Autodesk Inventor part; units mm, degrees
ref_plane "YZ Plane" through (0, 0, 0) normal (1, 0, 0) x (0, 1, 0)
ref_plane "XZ Plane" through (0, 0, 0) normal (0, 1, 0) x (-1, 0, 0)
ref_plane "XY Plane" through (0, 0, 0) normal (0, 0, 1) x (1, 0, 0)
sketch "Sketch1" plane through (0, 0, 0) normal (1, 0, 0) x (0, 1, 0)
  line L0 (0, 0) -> (120, 0)
  line L1 (100, -61.25) -> (95, -61.25)
  line L2 (95, -61.25) -> (95, -110)
  line L3 (95, -110) -> (0, -110)
  line L4 (0, -110) -> (0, -135)
  line L5 (0, -135) -> (10, -135)
  line L6 (10, -135) -> (10, -115)
  line L7 (10, -115) -> (100, -115)
  line L8 (100, -115) -> (100, -61.25)
  line L9 (0, -114) -> (2, -114)
  line L10 (2, -114) -> (2, -117)
  line L11 (2, -117) -> (0, -117)
  line L12 (0, -117) -> (0, -114)
  dimension "d1" = 270
  dimension "d2" = 220
  dimension "d3" = 230
  dimension "d4" = 122.5
  dimension "d5" = 10
  dimension "d6" = 5
  dimension "d7" = 100
  dimension "d21" = 228
  dimension "d22" = 3
  dimension "d24" = 2
revolve "Revolution1" add sketch "Sketch1" angle 360 about axis through (0, 0, 0) along (0, 1, 0) contours L8 L7 L6 L5 L4 L11 L10 L9 L3 L2 L1
sketch "Sketch2" plane through (0, 10, 0) normal (0, 1, 0) x (1, 0, 0)
  point P0 (0, 0)
  point P1 (0, 125)
  point P2 (-73.4732, 101.1271)
  point P3 (-118.8821, 38.6271)
  point P4 (-118.8821, -38.6271)
  point P5 (-73.4732, -101.1271)
  point P6 (0, -125)
  point P7 (73.4732, -101.1271)
  point P8 (118.8821, -38.6271)
  point P9 (118.8821, 38.6271)
  point P10 (73.4732, 101.1271)
  dimension "d9" = 125
  dimension "d12" = 360
hole "Hole1" at (0, 10, -125) at (-73.4732, 10, -101.1271) at (-118.8821, 10, -38.6271) at (-118.8821, 10, 38.6271) at (-73.4732, 10, 101.1271) at (0, 10, 125) at (73.4732, 10, 101.1271) at (118.8821, 10, 38.6271) at (118.8821, 10, -38.6271) at (73.4732, 10, -101.1271) direction (0, -1, 0) diameter 5.9 end through all counterbore diameter 10.2 counterbore depth 1.2
properties part number "Vibrometer Housing"
Read the model definition and answer for the solid it produces. Units are mm, in the model's axes. A direction names the side the tool comes from. Coordinates: 2 decimals unless noted, no trailing zeros. Write each loop counter-clockwise with the first axis right and the second up, starting at its lowest first coordinate (ties: lowest second). Pieces come first, ordered by that corner, then holes. Notation, with made-up numbers: (-21.5, -27.75) -> (-13.5, -27.75) arc R29 ccw to (-13.5, -6.75) -> close; hole circle Ø5 at (45.25, 17). An arc over 180 degrees is marked (long way). Return JSON: item names as keys, results as strings.
(1) Which of the six approach directions +Z, -Z, +X, -X, +Y, -Y give full straight-line access (tool end or side, diameter ignored) to faces 3 (the cylindrical face through (-59.793, 97.465, 13.278)), 4 (the flat face through (-71, 8.8, -99)), 5 (the cylindrical face through (43.66, 1.01, -105.31))?
Answers below:
{"face 3": "+Y, -Y", "face 4": "+Y", "face 5": "-Y"}
(2) The part is cut by section B-B on y = 42. Give the vertices of the cut face in (x, z).
Answers below:
{"outline": "circle Ø230 at (0, 0); hole circle Ø220 at (0, 0)"}
(3) The part is cut by section C-C on x = -55.5. Give the vertices of the cut face in (y, z).
Answers below:
{"outline": "(0, -123.06) -> (10, -123.06) -> (10, -100.72) -> (100, -100.72) -> (100, -25.91) -> (95, -25.91) -> (95, -94.97) -> (0, -94.97) -> (0, -99.58) -> (2, -99.58) -> (2, -103) -> (0, -103) -> close; (0, 94.97) -> (95, 94.97) -> (95, 25.91) -> (100, 25.91) -> (100, 100.72) -> (10, 100.72) -> (10, 123.06) -> (0, 123.06) -> (0, 103) -> (2, 103) -> (2, 99.58) -> (0, 99.58) -> close"}
(4) Consider line 1 along Z through (x, y) = (3, 46); line 2 along Z through (x, y) = (0, 98.9); line 3 along Y through (x, z) = (40.5, -117). Determine where each line is inside the solid, lowest interval first. Write a range as from..to.
Answers below:
{"line 1": "-114.96..-109.96, 109.96..114.96", "line 2": "-115..-61.25, 61.25..115", "line 3": "0..10"}
(5) Each of these flat-tipped pins is pushed along its axis until it touches: P1, Ø4, axis at y = 55.5, z = 31.5, coming from the +X side; P2, Ø13.5, axis at x = -73.47, z = 101.13, coming from the +Y side; P3, Ø4, axis at y = 31, z = -10.5, coming from the -X side. Where does it stop, or does it pass through?
Answers below:
{"P1": "x = 111.15", "P2": "y = 10", "P3": "x = -114.69"}
(6) For a pull along X with two mould halves and no side action, classify faces 1 (the flat face through (109, 10, -39)), 2 (the cylindrical face through (77.998, 9.392, -98.774)) as pulls with the +X half, pulls with the -X half, needs draft (parallel to the pull), parting line crosses it, or undercut.
Answers below:
{"face 1": "needs draft", "face 2": "undercut"}
(7) The part is cut by section A-A on z = 0. Give the vertices of the cut face in (x, y).
Answers below:
{"outline": "(-135, 0) -> (-117, 0) -> (-117, 2) -> (-114, 2) -> (-114, 0) -> (-110, 0) -> (-110, 95) -> (-61.25, 95) -> (-61.25, 100) -> (-115, 100) -> (-115, 10) -> (-135, 10) -> close; (61.25, 95) -> (110, 95) -> (110, 0) -> (114, 0) -> (114, 2) -> (117, 2) -> (117, 0) -> (135, 0) -> (135, 10) -> (115, 10) -> (115, 100) -> (61.25, 100) -> close"}
(8) The part is cut by section D-D on z = -77.5. Give the vertices of the cut face in (x, y), then the cut area to 3 significant figures.
Answers below:
{"outline": "(-110.54, 0) -> (-87.65, 0) -> (-87.65, 2) -> (-83.6, 2) -> (-83.6, 0) -> (-78.06, 0) -> (-78.06, 95) -> (78.06, 95) -> (78.06, 0) -> (83.6, 0) -> (83.6, 2) -> (87.65, 2) -> (87.65, 0) -> (110.54, 0) -> (110.54, 10) -> (84.96, 10) -> (84.96, 100) -> (-84.96, 100) -> (-84.96, 10) -> (-110.54, 10) -> close", "area": "2,660 mm^2"}
